Autodesk Inventor part; units mm, degrees
ref_plane "YZ Plane" through (0, 0, 0) normal (1, 0, 0) x (0, 1, 0)
ref_plane "XZ Plane" through (0, 0, 0) normal (0, 1, 0) x (-1, 0, 0)
ref_plane "XY Plane" through (0, 0, 0) normal (0, 0, 1) x (1, 0, 0)
sketch "Sketch1" plane through (0, 0, 0) normal (0, 1, 0) x (-1, 0, 0)
  circle A0 centre (0, 0) radius 1.05 construction
  arc A1 (-0.35, 1.2624) -> (-0.35, -1.2624) centre (0, 0) ccw
  circle A2 centre (0, 0) radius 4.5
  line L0 (0.35, 1.875) -> (-0.35, 1.875)
  line L1 (-0.35, 1.875) -> (-0.35, -1.875)
  line L2 (-0.35, -1.875) -> (0.35, -1.875)
  line L3 (0.35, -1.875) -> (0.35, 1.875)
  arc A3 (0.35, 1.2624) -> (-0.35, 1.2624) centre (0, 0) ccw
  arc A4 (0.35, -1.2624) -> (0.35, 1.2624) centre (0, 0) ccw
  arc A5 (-0.35, -1.2624) -> (0.35, -1.2624) centre (0, 0) ccw
  point P0 (0, 1.875)
  point P1 (0.35, 0)
  dimension "d1" = 2.1
  dimension "d3" = 9
  dimension "d18" = 0.26
  dimension "d19" = 0.7
  dimension "d20" = 3.75
extrude "Extrusion1" add sketch "Sketch1" along normal blind 3.5
sketch "Sketch4" plane through (0, 0, 0) normal (0, 0, 1) x (1, 0, 0)
  line L0 (-8.1, 20.5) -> (-8.1, 12.5)
  arc A0 (-8.1, 12.5) -> (8.1, 12.5) centre (0, 12.5) ccw
  line L1 (8.1, 12.5) -> (8.1, 20.5)
  line L2 (-6.1, 20.5) -> (-6.1, 18.1711)
  arc A1 (-6.1, 12.5) -> (-6.0523, 11.7389) centre (0, 12.5) ccw
  line L3 (6.1, 12.5) -> (6.1, 11.8289)
  line L4 (-8.1, 20.5) -> (-6.1, 20.5)
  line L5 (6.1, 20.5) -> (8.1, 20.5)
  line L6 (-0.35, 0) -> (0.35, 0)
  line L7 (4.5, 3.5) -> (-4.5, 3.5)
  arc A2 (-6.0523, 11.7389) -> (6.0523, 11.7389) centre (0, 15) ccw
  line L8 (-6.1, 18.1711) -> (-6.1, 11.8289)
  line L9 (-6.1, 11.8289) -> (-6.1, 12.5)
  line L10 (6.1, 11.8289) -> (6.1, 18.1711)
  line L11 (6.1, 18.1711) -> (6.1, 20.5)
  arc A3 (-6.1, 11.8289) -> (-6.0523, 11.7389) centre (0, 15) ccw
  arc A4 (6.1, 11.8289) -> (-6.1, 11.8289) centre (0, 15) ccw
  arc A5 (6.0523, 11.7389) -> (6.1, 11.8289) centre (0, 15) ccw
  arc A6 (6.0523, 11.7389) -> (6.1, 12.5) centre (0, 12.5) ccw
  arc A7 (-6.0523, 11.7389) -> (6.0523, 11.7389) centre (0, 12.5) ccw
  point P0 (0, 0)
  point P1 (0, 0)
  dimension "d23" = 2
  dimension "d24" = 9
  dimension "d25" = 8
  dimension "d26" = 13.75
  dimension "d27" = 2.5
  dimension "d36" = 12.2
extrude "Extrusion5" add sketch "Sketch4" along normal mid plane 9 contours L4 L2 A4 A3 A7 A5 L11 L5 L1 A0 L0
sketch "Sketch8" plane through (0, 3.5, 0) normal (0, 1, 0) x (1, 0, 0)
  circle A0 centre (0, 0) radius 4
  arc A1 (0.35, -1.2624) -> (0.35, 1.2624) centre (0, 0) ccw
  line L0 (0.35, 1.875) -> (0.35, 1.2624)
  line L1 (-0.35, 1.875) -> (0.35, 1.875)
  line L2 (-0.35, 1.2624) -> (-0.35, 1.875)
  arc A2 (-0.35, 1.2624) -> (-0.35, -1.2624) centre (0, 0) ccw
  line L3 (-0.35, -1.875) -> (-0.35, -1.2624)
  line L4 (0.35, -1.875) -> (-0.35, -1.875)
  line L5 (0.35, -1.2624) -> (0.35, -1.875)
  dimension "d33" = 8
extrude "Extrusion6" add sketch "Sketch8" along normal up to next
sketch "Sketch2" plane through (0, 3.5, 0) normal (0, 1, 0) x (1, 0, 0)
  circle A0 centre (0, 0) radius 1.31
  circle A1 centre (0, 0) radius 3.31
  dimension "d6" = 2
  dimension "d9" = 7.3
  dimension "d10" = 2
properties part number "LaserDiodeAdapterLarge" material "ABS Plastic"
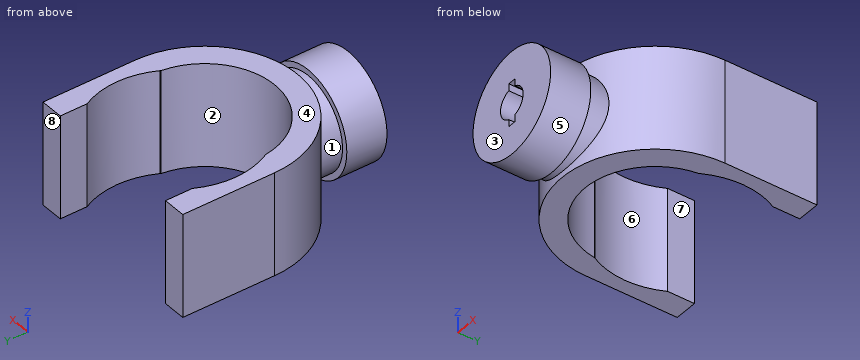
Design review of the part built by this model. Coordinates are the model's own, in mm. Face numbers are marked on the shaded views. A direction names the side the tool comes from. Round coordinates to 2 decimals unless told otherwise and drop trailing zeros. Write each loop counter-clockwise with the first axis right and the second up, starting at its lowest first coordinate (ties: lowest second). Pieces come first, ordered by that corner, then holes. Notation, with made-up numbers: (29, 27.5) - (37, 27.5) arc R21 ccw to (37, 33.5) - close; hole circle Ø10 at (23.25, 86.25). An arc over 180 degrees is marked (long way). Return JSON: item names as keys, results as strings. Group by question number.
Item 1: The part is to be moulded in two halves that separate along Y. For the marked faces 1, 2, 3 and 4, say which applies: pulls with the +Y half, pulls with the -Y half, needs draft (parallel to the pull), parting line crosses it, or undercut.
Item 2: We need section A-A on x = 0. Write out the cut boundary in (y, z) (3 decimals), and give its area (3 significant figures).
Item 3: Machinability: for the marked faces 5, 6, 7 and 8, which of the approach directions +Z, -Z, +X, -X, +Y, -Y give a long, thin tool a straight path to every point of the face, cutting with its end or side? Answer none if there is none.
Item 4: Insertion check: P1, Ø0.7, axis at y = 3, z = -1.5, coming from the -X side; P2, Ø5, axis at x = 1, z = 0.5, coming from the +Y side; P3, Ø0.7, axis at y = 2.5, z = 1.5, coming from the +X side. Each pin has a flat end and moves straight along its axis. Give the tip position at first contact, or say it passes through.
Item 5: We need section B-B on y = 15.25. Write out the cut boundary in (x, z).
Item 6: We need section D-D on z = 0. Write out the cut boundary in (x, y).
Item 7: For probe 1 along X at (y, z) = (14, 2.5); probe 2 along X at (y, z) = (7.5, 0.75); probe 3 along Y at (x, z) = (-4, 1.5), list the stretches that pass through material, from the lowest coordinate up. Write a range as [from, to].
Item 8: We need section C-C on y = 3.75. Write out the cut boundary in (x, z) (3 decimals).
Model answer:
{
 "1": {"face 1": "undercut", "face 2": "pulls with the +Y half", "face 3": "pulls with the -Y half", "face 4": "needs draft"},
 "2": {"outline": "(0, -4.5) - (3.5, -4.5) - (3.5, -4) - (4.4, -4) - (4.4, -4.5) - (6.4, -4.5) - (6.4, 4.5) - (4.4, 4.5) - (4.4, 4) - (3.5, 4) - (3.5, 4.5) - (0, 4.5) - (0, 1.875) - (4.4, 1.875) - (4.4, -1.875) - (0, -1.875) - close", "area": "40.2 mm²"},
 "3": {"face 5": "-Y", "face 6": "+Z, -Z", "face 7": "+Z, -Z, +Y", "face 8": "+Z, -Z, +X, -X, +Y"},
 "4": {"P1": "stops at x = -4.35", "P2": "stops at y = 7.5", "P3": "stops at x = 4.35"},
 "5": {"outline": "(-8.1, -4.5) - (-6.87, -4.5) - (-6.87, 4.5) - (-8.1, 4.5) - close; (6.87, -4.5) - (8.1, -4.5) - (8.1, 4.5) - (6.87, 4.5) - close"},
 "6": {"outline": "(-8.1, 12.5) arc R8.1 ccw to (-4, 5.46) - (-4, 3.5) - (-4.5, 3.5) - (-4.5, 0) - (-1.31, 0) - (-1.31, 4.51) arc R8.1 ccw to (1.31, 4.51) - (1.31, 0) - (4.5, 0) - (4.5, 3.5) - (4, 3.5) - (4, 5.46) arc R8.1 ccw to (8.1, 12.5) - (8.1, 20.5) - (6.1, 20.5) - (6.1, 18.17) arc R6.88 cw to (6.1, 11.83) arc R8.07 cw to (6.05, 11.74) arc R6.1 cw to (-6.05, 11.74) arc R5.99 cw to (-6.1, 11.83) arc R6.88 cw to (-6.1, 18.17) - (-6.1, 20.5) - (-8.1, 20.5) - close"},
 "7": {"probe 1": "x = [-8.1, -6.8], [6.8, 8.1]", "probe 2": "x = [-6.37, -3.49], [3.49, 6.37]", "probe 3": "y = [0, 3.5], [5.46, 7.89]"},
 "8": {"outline": "circle Ø8 at (0, 0); hole (-0.35, -1.875) - (0.35, -1.875) - (0.35, -1.262) arc R1.31 ccw to (0.35, 1.262) - (0.35, 1.875) - (-0.35, 1.875) - (-0.35, 1.262) arc R1.31 ccw to (-0.35, -1.262) - close"}
}
